CAD build for the part. Positions are in the model's coordinates, mm. Round coordinates to 2 decimals unless told otherwise and drop trailing zeros. Loops run counter-clockwise (first coordinate to the right, second up) from the corner with the lowest first, then second, coordinate; pieces in that order, holes last. Notation, with made-up numbers: (-17, 54.25) - (27, 54.25) arc R19 ccw to (27, 64.25) - close; hole circle Ø6 at (57.5, 70). An arc over 180 degrees is marked (long way). Use one line per item in the form item = value.
from build123d import *

# Parameters (mm, degrees)
SKETCH_1_W          = 100
SKETCH_1_H          = 40
EXTRUDE_1_DEPTH     = 3
SKETCH_2_R          = 1.5
CUT_EXTRUDE_1_DEPTH = 3
FILLET_1_R          = 1
CUT_EXTRUDE_2_DEPTH = 10
FILLET_2_R          = 1
SKETCH_4_R          = 1.5
CUT_EXTRUDE_3_DEPTH = 10


with BuildPart() as part:
    # 草图1 → 凸台-拉伸1 (new body)
    with BuildSketch(Plane(origin=(0, 0, 0), x_dir=(1, 0, 0), z_dir=(0, 1, 0))):
        Rectangle(SKETCH_1_W, SKETCH_1_H)
    extrude(amount=EXTRUDE_1_DEPTH)

    # 草图2 → 切除-拉伸1 (cut)
    with BuildSketch(Plane(origin=(0, 3, 0), x_dir=(1, 0, 0), z_dir=(0, 1, 0))):
        with Locations(Location((10, 17, 0), (0, 0, 270))):
            Circle(SKETCH_2_R)
        with Locations(Location((30, 17, 0), (0, 0, 270))):
            Circle(SKETCH_2_R)
    extrude(amount=-CUT_EXTRUDE_1_DEPTH, mode=Mode.SUBTRACT)

    # 圆角1
    fillet_1_edges = [part.edges().sort_by_distance(p)[0] for p in [
        (50, 1.5, 20),
        (-50, 1.5, 20),
        (-50, 1.5, -20),
        (50, 1.5, -20),
    ]]
    fillet(fillet_1_edges, radius=FILLET_1_R)

    # 草图3 → 切除-拉伸2 (cut)
    with BuildSketch(Plane(origin=(0, 3, 0), x_dir=(1, 0, 0), z_dir=(0, 1, 0))):
        Polygon((-29, 10.07179677), (-33, 17), (-41, 17), (-45, 10.07179677), (-41, 3.143593539), (-33, 3.143593539), align=None)
        Polygon((-11.503632276, -10.07179677), (-15.503632276, -3.143593539), (-23.503632276, -3.143593539), (-27.503632276, -10.07179677), (-23.503632276, -17), (-15.503632276, -17), align=None)
        Polygon((5.992735447, 10.07179677), (1.992735447, 17), (-6.007264553, 17), (-10.007264553, 10.07179677), (-6.007264553, 3.143593539), (1.992735447, 3.143593539), align=None)
        Polygon((23.489103171, -10.07179677), (19.489103171, -3.143593539), (11.489103171, -3.143593539), (7.489103171, -10.07179677), (11.489103171, -17), (19.489103171, -17), align=None)
    extrude(amount=-CUT_EXTRUDE_2_DEPTH, mode=Mode.SUBTRACT)

    # 圆角2
    fillet_2_edges = [part.edges().sort_by_distance(p)[0] for p in [
        (-11.503632276, 1.5, 10.07179677),
        (-15.503632276, 1.5, 17),
        (-23.503632276, 1.5, 17),
        (-27.503632276, 1.5, 10.07179677),
        (-23.503632276, 1.5, 3.143593539),
        (-15.503632276, 1.5, 3.143593539),
        (23.489103171, 1.5, 10.07179677),
        (19.489103171, 1.5, 17),
        (11.489103171, 1.5, 17),
        (7.489103171, 1.5, 10.07179677),
        (11.489103171, 1.5, 3.143593539),
        (19.489103171, 1.5, 3.143593539),
        (-29, 1.5, -10.07179677),
        (-33, 1.5, -3.143593539),
        (-41, 1.5, -3.143593539),
        (-45, 1.5, -10.07179677),
        (-41, 1.5, -17),
        (-33, 1.5, -17),
        (5.992735447, 1.5, -10.07179677),
        (1.992735447, 1.5, -3.143593539),
        (-6.007264553, 1.5, -3.143593539),
        (-10.007264553, 1.5, -10.07179677),
        (-6.007264553, 1.5, -17),
        (1.992735447, 1.5, -17),
    ]]
    fillet(fillet_2_edges, radius=FILLET_2_R)

    # 草图4 → 切除-拉伸3 (cut)
    with BuildSketch(Plane(origin=(0, 3, 0), x_dir=(1, 0, 0), z_dir=(0, 1, 0))):
        with Locations(Location((-45, -15, 0), (0, 0, 270))):
            Circle(SKETCH_4_R)
        with Locations(Location((45, -15, 0), (0, 0, 270))):
            Circle(SKETCH_4_R)
    extrude(amount=-CUT_EXTRUDE_3_DEPTH, mode=Mode.SUBTRACT)


solid = part.part
1) Slice it at D-D (z = 15). Write the cut outline in (x, y), plus the area to 3 significant figures.
Report:
outline = (-50, 0) - (-46.5, 0) - (-46.5, 3) - (-50, 3) - close; (-43.5, 0) - (-24.66, 0) - (-24.66, 3) - (-43.5, 3) - close; (-14.35, 0) - (10.33, 0) - (10.33, 3) - (-14.35, 3) - close; (20.64, 0) - (43.5, 0) - (43.5, 3) - (20.64, 3) - close; (46.5, 0) - (50, 0) - (50, 3) - (46.5, 3) - close
area = 220 mm^2
2) Flat gauge pin, fed straight in: pin 1 (5 mm diameter, centred on x = 30, z = -17, fed in from -Y). Where does the tip first touch, or does it go through?
Report:
pin_1 = 0
3) Slice it at C-C (z = -6). Write the cut outline in (x, y), plus the area to 3 significant figures.
Report:
outline = (-50, 0) - (-42.65, 0) - (-42.65, 3) - (-50, 3) - close; (-31.35, 0) - (-7.66, 0) - (-7.66, 3) - (-31.35, 3) - close; (3.64, 0) - (50, 0) - (50, 3) - (3.64, 3) - close
area = 232 mm^2
4) Drill centre lines: probe 1 along Z at (x, y) = (-36.5, 1.8); probe 2 along X at (y, z) = (0.3, 5.5); probe 3 along X at (y, z) = (0.8, 15.5). Where is each one in solid material? Low to high.
Report:
probe_1 = -20 to -17, -3.14 to 20
probe_2 = -50 to -24.86, -14.14 to 10.13, 20.85 to 50
probe_3 = -50 to -46.41, -43.59 to -24.37, -14.64 to 10.62, 20.36 to 43.59, 46.41 to 50
5) Slice it at B-B (x = 10). Write the cut outline in (y, z), plus the area to 3 significant figures.
Report:
outline = (0, -20) - (3, -20) - (3, -18.5) - (0, -18.5) - close; (0, -15.5) - (3, -15.5) - (3, 5.72) - (0, 5.72) - close; (0, 14.42) - (3, 14.42) - (3, 20) - (0, 20) - close
area = 84.9 mm^2
6) Two-plate mould, pull along X, no slides. Class faces 1 (the cylindrical face through (-46.464, 1.521, 14.675)), 2 (the flat face through (-2, 2, -3.144)), 3 (the flat face through (-1, 0, 0)), 4 (the flat face through (-50, 1, 0)): +X half, -X half, draft (parallel to the pull), parting line (faces both ways), or undercut.
Report:
face_1 = undercut
face_2 = undercut
face_3 = draft
face_4 = -X half
7) Slice it at A-A (x = 45). Write the cut outline in (y, z).
Report:
outline = (0, -20) - (3, -20) - (3, 13.5) - (0, 13.5) - close; (0, 16.5) - (3, 16.5) - (3, 20) - (0, 20) - close
